Input: part model. Units: mm. Frame: model coordinates. A direction names the side the tool comes from. Coordinates: 2 decimals unless noted, no trailing zeros. Order: outer loops, then holes, each group sorted by start corner. A loop starts at its lowest first (then second) coordinate and runs counter-clockwise, first axis right, second up. Notation, with made-up numbers: M -15,54.5 L 35,54.5 A21 ccw 35,73.5 Z; hole C 15.5,-20.5 d9. An arc over 180 degrees is marked long. Answer in a Markdown table with one row per item.
from build123d import *

# Parameters (mm, degrees)
SKETCH1_W           = 47
SKETCH1_H           = 16.3
SKETCH1_R           = 1.9
BOSS_EXTRUDE1_DEPTH = 3
SKETCH2_R           = 3.25
BOSS_EXTRUDE2_DEPTH = 10
FILLET1_R           = 1
FILLET2_R           = 2


with BuildPart() as part:
    # Sketch1 → Boss-Extrude1 (new body)
    with BuildSketch(Plane.XY):
        Rectangle(SKETCH1_W, SKETCH1_H)
        with Locations((19.5, 5)):
            Circle(SKETCH1_R, mode=Mode.SUBTRACT)
        with Locations((19.5, -5)):
            Circle(SKETCH1_R, mode=Mode.SUBTRACT)
    extrude(amount=BOSS_EXTRUDE1_DEPTH)

    # Sketch2 → Boss-Extrude2 (add)
    with BuildSketch(Plane.XY):
        with Locations((-15.3, 0)):
            Circle(SKETCH2_R)
    extrude(amount=BOSS_EXTRUDE2_DEPTH)

    # Fillet1
    fillet1_edges = [part.edges().sort_by_distance(p)[0] for p in [
        (-23.5, 0, 3),
        (0, -8.15, 3),
        (23.5, 0, 3),
        (0, -8.15, 0),
        (-23.5, 0, 0),
        (0, 8.15, 0),
        (23.5, 0, 0),
        (0, 8.15, 3),
    ]]
    fillet(fillet1_edges, radius=FILLET1_R)

    # Fillet2
    # the kernel refuses this fillet: 2 mm, written as the material it takes off along each edge
    with BuildSketch(Plane(origin=(-21.5, -6.15, 0), x_dir=(0, -1, 0), z_dir=(1, 0, 0))) as fillet2_piece_1:
        with BuildLine():
            CenterArc((1, -1), 1, 0, 90)
            Line((2, -1), (2, 0))
            Line((2, 0), (1, 0))
        make_face()
    revolve(axis=Axis((-21.5, -6.15, 0), (0, 0, -1)), revolution_arc=90, mode=Mode.SUBTRACT)
    with BuildSketch(Plane(origin=(-21.5, 6.15, 0), x_dir=(-1, 0, 0), z_dir=(0, -1, 0))) as fillet2_piece_2:
        with BuildLine():
            CenterArc((1, -1), 1, 0, 90)
            Line((2, -1), (2, 0))
            Line((2, 0), (1, 0))
        make_face()
    revolve(axis=Axis((-21.5, 6.15, 0), (0, 0, -1)), revolution_arc=90, mode=Mode.SUBTRACT)
    with BuildSketch(Plane(origin=(21.5, -6.15, 0), x_dir=(1, 0, 0), z_dir=(0, 1, 0))) as fillet2_piece_3:
        with BuildLine():
            CenterArc((1, -1), 1, 0, 90)
            Line((2, -1), (2, 0))
            Line((2, 0), (1, 0))
        make_face()
    revolve(axis=Axis((21.5, -6.15, 0), (0, 0, -1)), revolution_arc=90, mode=Mode.SUBTRACT)
    with BuildSketch(Plane(origin=(21.5, 6.15, 0), x_dir=(0, 1, 0), z_dir=(-1, 0, 0))) as fillet2_piece_4:
        with BuildLine():
            CenterArc((1, -1), 1, 0, 90)
            Line((2, -1), (2, 0))
            Line((2, 0), (1, 0))
        make_face()
    revolve(axis=Axis((21.5, 6.15, 0), (0, 0, -1)), revolution_arc=90, mode=Mode.SUBTRACT)
    with BuildSketch(Plane(origin=(21.5, -6.15, 3), x_dir=(0, -1, 0), z_dir=(-1, 0, 0))) as fillet2_piece_5:
        with BuildLine():
            CenterArc((1, -1), 1, 0, 90)
            Line((2, -1), (2, 0))
            Line((2, 0), (1, 0))
        make_face()
    revolve(axis=Axis((21.5, -6.15, 3), (0, 0, 1)), revolution_arc=90, mode=Mode.SUBTRACT)
    with BuildSketch(Plane(origin=(-21.5, -6.15, 3), x_dir=(-1, 0, 0), z_dir=(0, 1, 0))) as fillet2_piece_6:
        with BuildLine():
            CenterArc((1, -1), 1, 0, 90)
            Line((2, -1), (2, 0))
            Line((2, 0), (1, 0))
        make_face()
    revolve(axis=Axis((-21.5, -6.15, 3), (0, 0, 1)), revolution_arc=90, mode=Mode.SUBTRACT)
    with BuildSketch(Plane(origin=(21.5, 6.15, 3), x_dir=(1, 0, 0), z_dir=(0, -1, 0))) as fillet2_piece_7:
        with BuildLine():
            CenterArc((1, -1), 1, 0, 90)
            Line((2, -1), (2, 0))
            Line((2, 0), (1, 0))
        make_face()
    revolve(axis=Axis((21.5, 6.15, 3), (0, 0, 1)), revolution_arc=90, mode=Mode.SUBTRACT)
    with BuildSketch(Plane(origin=(-21.5, 6.15, 3), x_dir=(0, 1, 0), z_dir=(1, 0, 0))) as fillet2_piece_8:
        with BuildLine():
            CenterArc((1, -1), 1, 0, 90)
            Line((2, -1), (2, 0))
            Line((2, 0), (1, 0))
        make_face()
    revolve(axis=Axis((-21.5, 6.15, 3), (0, 0, 1)), revolution_arc=90, mode=Mode.SUBTRACT)
    with BuildSketch(Plane(origin=(23.5, 8.15, 0), x_dir=(-1, 0, 0), z_dir=(0, 0, 1)), Plane(origin=(23.5, -8.15, 0), x_dir=(0, 1, 0), z_dir=(0, 0, 1))) as fillet2_piece_9:
        with BuildLine():
            CenterArc((FILLET2_R, FILLET2_R), FILLET2_R, 180, 90)
            Line((0, FILLET2_R), (0, 0))
            Line((0, 0), (FILLET2_R, 0))
        make_face()
    extrude(amount=3, mode=Mode.SUBTRACT)
    with BuildSketch(Plane(origin=(-23.5, -8.15, 0), x_dir=(0, 1, 0), z_dir=(0, 0, 1)), Plane(origin=(-23.5, 8.15, 0), x_dir=(1, 0, 0), z_dir=(0, 0, 1))) as fillet2_piece_10:
        with BuildLine():
            CenterArc((FILLET2_R, -FILLET2_R), FILLET2_R, 90, 90)
            Line((0, -FILLET2_R), (0, 0))
            Line((0, 0), (FILLET2_R, 0))
        make_face()
    extrude(amount=3, mode=Mode.SUBTRACT)


solid = part.part
1) Cut plane C-C, the plane x = 4. Output: boundary loops of the cut face in (y, z).
Resolved:
| item | result |
|---|---|
| outline | M -8.15,1 A1 ccw -7.15,0 L 7.15,0 A1 ccw 8.15,1 L 8.15,2 A1 ccw 7.15,3 L -7.15,3 A1 ccw -8.15,2 Z |
2) Cut plane B-B, the plane z = 1.5. Output: boundary loops of the cut face in (x, y).
Resolved:
| item | result |
|---|---|
| outline | M -23.5,-6.15 A2 ccw -21.5,-8.15 L 21.5,-8.15 A2 ccw 23.5,-6.15 L 23.5,6.15 A2 ccw 21.5,8.15 L -21.5,8.15 A2 ccw -23.5,6.15 Z; hole C 19.5,-5 d3.8; hole C 19.5,5 d3.8 |
3) Material intervals for probe 1 along Y at (x, z) = (19.5, 1.1); probe 2 along Y at (x, z) = (19.5, 2.2); probe 3 along Z at (x, y) = (14, -0.25), sorted ascending.
Resolved:
| item | result |
|---|---|
| probe 1 | y = -8.15 to -6.9, -3.1 to 3.1, 6.9 to 8.15 |
| probe 2 | y = -8.13 to -6.9, -3.1 to 3.1, 6.9 to 8.13 |
| probe 3 | z = 0 to 3 |
4) Cut plane D-D, the plane y = 0. Output: boundary loops of the cut face in (x, z), and give its area (3 significant figures).
Resolved:
| item | result |
|---|---|
| outline | M -23.5,1 A1 ccw -22.5,0 L 22.5,0 A1 ccw 23.5,1 L 23.5,2 A1 ccw 22.5,3 L -12.05,3 L -12.05,10 L -18.55,10 L -18.55,3 L -22.5,3 A1 ccw -23.5,2 Z |
| area | 186 mm2 |
5) Mould query, pull axis X, two halves, no side actions, for faces 3 (the face through (0.301, 7.865, 2.699)), 4 (the face through (18.1, -3.716, 1.479)), 5 (the face through (18.1, 6.284, 1.479)), 6 (the face through (-22.9, 7.58, 1.49)). Classes: +X half, -X half, draft (parallel to the pull), parting line (faces both ways), or undercut.
Resolved:
| item | result |
|---|---|
| face 3 | draft |
| face 4 | undercut |
| face 5 | undercut |
| face 6 | -X half |
6) Cut plane A-A, the plane y = -5. Output: boundary loops of the cut face in (x, z), and give its area (3 significant figures).
Resolved:
| item | result |
|---|---|
| outline | M -23.5,1 A1 ccw -22.5,0 L 17.6,0 L 17.6,3 L -22.5,3 A1 ccw -23.5,2 Z; M 21.4,0 L 22.5,0 A1 ccw 23.5,1 L 23.5,2 A1 ccw 22.5,3 L 21.4,3 Z |
| area | 129 mm2 |
7) Reachability of faces 1 (the face through (-12.2, 0.98, 6.45)), 2 (the face through (23.5, -0.1, 1.5)) from +Z, -Z, +X, -X, +Y, -Y: full face, straight path, thin tool, end or side. Return the list, or none.
Resolved:
| item | result |
|---|---|
| face 1 | +Z |
| face 2 | +Z, -Z, +X, +Y, -Y |
8) Contact query for flat-ended pins moving along their axis: pin 1 (6 mm diameter, centred on y = -4.5, z = 5, fed in from -X); pin 2 (3.5 mm diameter, centred on x = 19.5, y = 5, fed in from -Z); pin 3 (3 mm diameter, centred on x = -0.5, y = 4, fed in from +Z). Output: stop coordinate, or through.
Resolved:
| item | result |
|---|---|
| pin 1 | stops at x = -23.5 |
| pin 2 | passes through |
| pin 3 | stops at z = 3 |
